```python
from build123d import *

# Parameters (mm, degrees)
F1_DEPTH = 30
F0_R     = 2.5
F2_DEPTH = 2
F3_R     = 3
F4_DEPTH = 2
F5_R     = 3
F6_DEPTH = 2


with BuildPart() as f1:
    # F0 (on Front) → F1 (new body)
    with BuildSketch(Plane.XZ):
        with BuildLine():
            Line((40, -43), (40, 43))
            Line((40, 43), (-40, 43))
            Line((-40, 43), (-40, -43))
            ThreePointArc((-40, -43), (0, -73.5773), (40, -43))
        make_face()
        with BuildLine():
            Line((-38, -29), (-38, 41))
            Line((-38, 41), (12, 41))
            Line((12, 41), (18, 41))
            Line((18, 41), (38, 41))
            Line((38, 41), (38, -35.250901))
            ThreePointArc((38, -35.250901), (-3.125451, -70.125451), (-38, -29))
        make_face(mode=Mode.SUBTRACT)
    extrude(amount=F1_DEPTH)

    # F0 (on Front) → F2 (join)
    with BuildSketch(Plane.XZ):
        with BuildLine():
            Line((12, 41), (-38, 41))
            Line((-38, 41), (-38, -29))
            ThreePointArc((-38, -29), (-3.125451, -70.125451), (38, -35.250901))
            Line((38, -35.250901), (38, 41))
            Line((38, 41), (18, 41))
            Line((18, 41), (18, -7))
            Line((18, -7), (12, -7))
            Line((12, -7), (12, 41))
        make_face()
        with Locations((-13.079933, -4.567117)):
            Circle(F0_R, mode=Mode.SUBTRACT)
        with Locations((-5.079933, -4.567117)):
            Circle(F0_R, mode=Mode.SUBTRACT)
        with Locations((-13.079933, 37.432883)):
            Circle(F0_R, mode=Mode.SUBTRACT)
        with Locations((-5.079933, 37.432883)):
            Circle(F0_R, mode=Mode.SUBTRACT)
    extrude(amount=F2_DEPTH)

    # F3 (on face) → F4 (join)
    with BuildSketch(Plane.YZ.offset(40)):
        with BuildLine():
            Line((0, 27), (0, 3))
            ThreePointArc((0, 3), (12, 15), (0, 27))
        make_face()
        with Locations((5, 15)):
            Circle(F3_R, mode=Mode.SUBTRACT)
        with BuildLine():
            Line((0, -19), (0, -43))
            ThreePointArc((0, -43), (12, -31), (0, -19))
        make_face()
        with Locations((5, -31)):
            Circle(F3_R, mode=Mode.SUBTRACT)
    extrude(amount=-F4_DEPTH)

    # F5 (on face) → F6 (join)
    with BuildSketch(Plane(origin=(-40, 0, 0), x_dir=(0, -1, 0), z_dir=(-1, 0, 0))):
        with BuildLine():
            Line((0, -43), (0, -19))
            ThreePointArc((0, -19), (-12, -31), (0, -43))
        make_face()
        with Locations((-5, -31)):
            Circle(F5_R, mode=Mode.SUBTRACT)
        with BuildLine():
            Line((0, 3), (0, 27))
            ThreePointArc((0, 27), (-12, 15), (0, 3))
        make_face()
        with Locations((-4.808913, 14.980538)):
            Circle(F5_R, mode=Mode.SUBTRACT)
    extrude(amount=-F6_DEPTH)


solid = f1.part
```
Geometry check sheet. Reference: the model listing, model coordinates, mm. A direction names the side the tool comes from. Round coordinates to 2 decimals unless told otherwise and drop trailing zeros. Write each loop counter-clockwise with the first axis right and the second up, starting at its lowest first coordinate (ties: lowest second). Pieces come first, ordered by that corner, then holes. Notation, with made-up numbers: (35.5, 5.25) -> (40.5, 5.25) arc R20 ccw to (40.5, 44.25) -> close; hole circle Ø5 at (36.5, 66). An arc over 180 degrees is marked (long way). Put each result on its own line as item: value.
1) Cross-section at B-B, the plane z = 7.5. Enter the section's corners in (x, y), plus the area to 3 significant figures.
Recorded:
outline: (-40, -30) -> (-38, -30) -> (-38, -2) -> (12, -2) -> (12, 0) -> (-38, 0) -> (-38, 9.37) -> (-40, 9.37) -> close; (18, -2) -> (38, -2) -> (38, -30) -> (40, -30) -> (40, 9.37) -> (38, 9.37) -> (38, 0) -> (18, 0) -> close
area: 297 mm2
2) Thickness scan on probe 1 along Z at (x, y) = (-38.95, 5); probe 2 along Z at (x, y) = (27, -24.5); probe 3 along Y at (x, z) = (7, -2). Record the ranges inside material, lowest first. Write a range as from..to.
Recorded:
probe 1: z = -41.91..-34, -28..-20.09, 4.09..11.99, 17.97..25.91
probe 2: z = -63.58..-59.05, 41..43
probe 3: y = -2..0
3) Depth check by flat-ended pin: P1, Ø24, axis at x = -12.5, z = -7, coming from the +Y side. Enter the tip coordinate at first touch or a pass-through.
Recorded:
P1: stops at y = 0
4) Access from +Z, -Z, +X, -X, +Y, -Y to the whole of each face (thin tool, end or side, straight path). Record for faces 4 (the face through (-1, -2, -14)), 5 (the face through (39.01, 4.35, 12.07)), 6 (the face through (38, 3, -28)).
Recorded:
face 4: -Y
face 5: +X
face 6: +Z, -Z, +Y
5) Release check for a two-part mould opening along X. For faces 1 (the face through (-7.578, -0.986, -4.457)), 2 (the face through (-39, 12, 15)), 3 (the face through (-40, -13, 1)) record: pulls with the +X half, pulls with the -X half, needs draft (parallel to the pull), parting line crosses it, or undercut.
Recorded:
face 1: undercut
face 2: needs draft
face 3: pulls with the -X half
6) Cross-section at D-D, the plane y = 5. Give the number of separate pieces and of enclosed holes in the cut face, plus the area to 3 significant figures.
Recorded:
separate pieces: 8
enclosed holes: 0
area: 127 mm2
7) Cross-section at C-C, the plane z = -31. Enter the section's corners in (x, y).
Recorded:
outline: (-40, -30) -> (-38.11, -30) -> (-38.11, -2) -> (38, -2) -> (38, -30) -> (40, -30) -> (40, 2) -> (38, 2) -> (38, 0) -> (-38, 0) -> (-38, 2) -> (-40, 2) -> close; (-40, 8) -> (-38, 8) -> (-38, 12) -> (-40, 12) -> close; (38, 8) -> (40, 8) -> (40, 12) -> (38, 12) -> close
